from build123d import *

# Parameters (mm, degrees)
MODEL_R         = 1.5
MODEL_R_2       = 1.6
MODEL_R_3       = 2
MODEL_R_4       = 10
MODEL_R_5       = 2.5
MODEL_W         = 19
MODEL_H         = 13
EXTRUDE_1_DEPTH = 3


with BuildPart() as part:
    # Model → 凸台-拉伸1 (new body)
    with BuildSketch(Plane.XY):
        with BuildLine():
            Line((5, 120), (398, 120))
            ThreePointArc((398, 120), (401.535533906, 118.535533906), (403, 115))
            Line((403, 115), (403, -115))
            ThreePointArc((403, -115), (401.535533906, -118.535533906), (398, -120))
            Line((398, -120), (5, -120))
            ThreePointArc((5, -120), (1.464466094, -118.535533906), (0, -115))
            Line((0, -115), (0, 115))
            ThreePointArc((0, 115), (1.464466094, 118.535533906), (5, 120))
        make_face()
        with Locations((17, 95.5)):
            Circle(MODEL_R, mode=Mode.SUBTRACT)
        with Locations((29, 95.5)):
            Circle(MODEL_R, mode=Mode.SUBTRACT)
        with Locations((47, 95.5)):
            Circle(MODEL_R, mode=Mode.SUBTRACT)
        with Locations((59, 95.5)):
            Circle(MODEL_R, mode=Mode.SUBTRACT)
        with Locations((17, -95.5)):
            Circle(MODEL_R, mode=Mode.SUBTRACT)
        with Locations((29, -95.5)):
            Circle(MODEL_R, mode=Mode.SUBTRACT)
        with Locations((47, -95.5)):
            Circle(MODEL_R, mode=Mode.SUBTRACT)
        with Locations((59, -95.5)):
            Circle(MODEL_R, mode=Mode.SUBTRACT)
        with Locations((4, 109.5)):
            Circle(MODEL_R, mode=Mode.SUBTRACT)
        with Locations((16, 109.5)):
            Circle(MODEL_R, mode=Mode.SUBTRACT)
        with Locations((4, -109.5)):
            Circle(MODEL_R, mode=Mode.SUBTRACT)
        with Locations((16, -109.5)):
            Circle(MODEL_R, mode=Mode.SUBTRACT)
        with Locations((362, 109.5)):
            Circle(MODEL_R, mode=Mode.SUBTRACT)
        with Locations((374, 109.5)):
            Circle(MODEL_R, mode=Mode.SUBTRACT)
        with Locations((362, -109.5)):
            Circle(MODEL_R, mode=Mode.SUBTRACT)
        with Locations((374, -109.5)):
            Circle(MODEL_R, mode=Mode.SUBTRACT)
        with Locations((361, 32)):
            Circle(MODEL_R_2, mode=Mode.SUBTRACT)
        with Locations((393, 32)):
            Circle(MODEL_R_2, mode=Mode.SUBTRACT)
        with Locations((393, -32)):
            Circle(MODEL_R_2, mode=Mode.SUBTRACT)
        with Locations((361, -32)):
            Circle(MODEL_R_2, mode=Mode.SUBTRACT)
        with Locations((188, 98)):
            Circle(MODEL_R_3, mode=Mode.SUBTRACT)
        with Locations((138, 98)):
            Circle(MODEL_R_3, mode=Mode.SUBTRACT)
        with Locations((254, 109.5)):
            Circle(MODEL_R, mode=Mode.SUBTRACT)
        with Locations((242, 109.5)):
            Circle(MODEL_R, mode=Mode.SUBTRACT)
        with Locations((188, -98)):
            Circle(MODEL_R_3, mode=Mode.SUBTRACT)
        with Locations((138, -98)):
            Circle(MODEL_R_3, mode=Mode.SUBTRACT)
        with Locations((138, -28)):
            Circle(MODEL_R_3, mode=Mode.SUBTRACT)
        with Locations((188, -28)):
            Circle(MODEL_R_3, mode=Mode.SUBTRACT)
        with Locations((295, 37)):
            Circle(MODEL_R_4, mode=Mode.SUBTRACT)
        with Locations((285, 51.5)):
            Circle(MODEL_R_5, mode=Mode.SUBTRACT)
        with Locations((305, 51.5)):
            Circle(MODEL_R_5, mode=Mode.SUBTRACT)
        with Locations((256, 18.5)):
            Circle(MODEL_R, mode=Mode.SUBTRACT)
        with Locations((246, 18.5)):
            Circle(MODEL_R, mode=Mode.SUBTRACT)
        with Locations((256, -18.5)):
            Circle(MODEL_R, mode=Mode.SUBTRACT)
        with Locations((246, -18.5)):
            Circle(MODEL_R, mode=Mode.SUBTRACT)
        with Locations((95, 60)):
            Circle(MODEL_R_4, mode=Mode.SUBTRACT)
        with Locations((105, 72.5)):
            Circle(MODEL_R_5, mode=Mode.SUBTRACT)
        with Locations((85, 72.5)):
            Circle(MODEL_R_5, mode=Mode.SUBTRACT)
        with Locations((95, -60)):
            Circle(MODEL_R_4, mode=Mode.SUBTRACT)
        with Locations((105, -72.5)):
            Circle(MODEL_R_5, mode=Mode.SUBTRACT)
        with Locations((85, -72.5)):
            Circle(MODEL_R_5, mode=Mode.SUBTRACT)
        with Locations((134, 109.5)):
            Circle(MODEL_R, mode=Mode.SUBTRACT)
        with Locations((122, 109.5)):
            Circle(MODEL_R, mode=Mode.SUBTRACT)
        with Locations((287, 10)):
            Circle(MODEL_R_3, mode=Mode.SUBTRACT)
        with Locations((303, 10)):
            Circle(MODEL_R_3, mode=Mode.SUBTRACT)
        with Locations((303, -10)):
            Circle(MODEL_R_3, mode=Mode.SUBTRACT)
        with Locations((287, -10)):
            Circle(MODEL_R_3, mode=Mode.SUBTRACT)
        with Locations((55.030468906, 71.000464285)):
            Circle(MODEL_R_3, mode=Mode.SUBTRACT)
        with Locations((71.030468906, 71.000464285)):
            Circle(MODEL_R_3, mode=Mode.SUBTRACT)
        with Locations((55.030468906, -71.000464285)):
            Circle(MODEL_R_3, mode=Mode.SUBTRACT)
        with Locations((71.030468906, -71.000464285)):
            Circle(MODEL_R_3, mode=Mode.SUBTRACT)
        with Locations((254, -109.5)):
            Circle(MODEL_R, mode=Mode.SUBTRACT)
        with Locations((242, -109.5)):
            Circle(MODEL_R, mode=Mode.SUBTRACT)
        with Locations((134, -109.5)):
            Circle(MODEL_R, mode=Mode.SUBTRACT)
        with Locations((122, -109.5)):
            Circle(MODEL_R, mode=Mode.SUBTRACT)
        with Locations((267.106872725, 18.5)):
            Circle(MODEL_R_5, mode=Mode.SUBTRACT)
        with Locations((234.893127275, 18.5)):
            Circle(MODEL_R_5, mode=Mode.SUBTRACT)
        with Locations((267.106872725, -18.5)):
            Circle(MODEL_R_5, mode=Mode.SUBTRACT)
        with Locations((234.893127275, -18.5)):
            Circle(MODEL_R_5, mode=Mode.SUBTRACT)
        with Locations((295, 66)):
            Rectangle(MODEL_W, MODEL_H, mode=Mode.SUBTRACT)
    extrude(amount=EXTRUDE_1_DEPTH)


solid = part.part
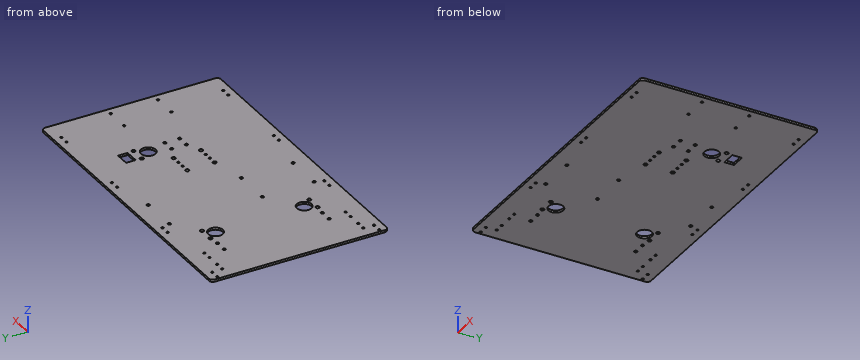
Here's how the part is built. I have some questions about the finished solid (model axes, mm). Give positions to 0.01 mm unless a question says otherwise; leave off trailing zeros. Order: outer loops, then holes, each group sorted by start corner. A loop starts at its lowest first (then second) coordinate and runs counter-clockwise, first axis right, second up. Notation, with made-up numbers: (-7, -11.75) -> (11, -11.75) arc R7 ccw to (11, -3.75) -> close; hole circle Ø9 at (-29.5, 70.5). An arc over 180 degrees is marked (long way). One line per item, written item: value. Start each with the question number.
1. Will this pin go through, and if not, where does the flat tip stop? pin 1 Ø2.5 at (x, y) = (122, -109.5) entering from -Z.
2. Imagine slicing it at A-A, the plane x = 295. List the corners of the cut face in (y, z) for me, plus the area to 3 significant figures.
3. Imagine slicing it at C-C, the plane z = 1.9. Count the separate pieces of the cut face and the enclosed holes in it, plus the area to 3 significant figures.
4. Imagine slicing it at B-B, the plane y = -60. List the corners of the cut face in (x, z) for me.
5. I need wall thicknesses on probe 1 along Y at (x, z) = (254, 0.85); probe 2 along Y at (x, z) = (94, 0.95); probe 3 along X at (y, z) = (-33, 1.4). Which ranges of each line are inside material? Lowest first, please. Write a range as from..to.
Values follow:
1. pin 1: passes through
2. outline: (-120, 0) -> (27, 0) -> (27, 3) -> (-120, 3) -> close; (47, 0) -> (59.5, 0) -> (59.5, 3) -> (47, 3) -> close; (72.5, 0) -> (120, 0) -> (120, 3) -> (72.5, 3) -> close
2. area: 621 mm2
3. separate pieces: 1
3. enclosed holes: 60
3. area: 94,900 mm2
4. outline: (0, 0) -> (85, 0) -> (85, 3) -> (0, 3) -> close; (105, 0) -> (403, 0) -> (403, 3) -> (105, 3) -> close
5. probe 1: y = -120..-111, -108..108, 111..120
5. probe 2: y = -120..-69.95, -50.05..50.05, 69.95..120
5. probe 3: x = 0..359.75, 362.25..391.75, 394.25..403
